For this review, take the finished solid that the model builds, in its own axes (mm). Round coordinates to 2 decimals unless told otherwise and drop trailing zeros. Write each loop counter-clockwise with the first axis right and the second up, starting at its lowest first coordinate (ties: lowest second). Pieces come first, ordered by that corner, then holes. Notation, with made-up numbers: (42.5, 59.5) -> (92.5, 59.5) arc R28 cw to (92.5, 78.5) -> close; hole circle Ø4 at (-3, -30). An arc over 180 degrees is marked (long way). Answer in a Markdown table with one row per item. Add a question column.
```python
from build123d import *

# Parameters (mm, degrees)
SKETCH1_W                                   = 50.5
SKETCH1_H                                   = 51.5
SKETCH1_R                                   = 1.775
BOSS_EXTRUDE1_DEPTH                         = 3.5
CSK_FOR_10_FLAT_HEAD_SOCKET_CAP_SCR_2_COUNT = 2
CSK_FOR_10_FLAT_HEAD_SOCKET_CAP_SCR_2_PITCH = 20


with BuildPart() as part:
    # Sketch1 → Boss-Extrude1 (new body)
    with BuildSketch(Plane(origin=(0, 0, 0), x_dir=(1, 0, 0), z_dir=(0, 1, 0))):
        Rectangle(SKETCH1_W, SKETCH1_H)
        with Locations(Location((-19.475, 19.975, 0), (0, 0, 270))):
            Circle(SKETCH1_R, mode=Mode.SUBTRACT)
        with Locations(Location((19.475, 19.975, 0), (0, 0, 270))):
            Circle(SKETCH1_R, mode=Mode.SUBTRACT)
        with Locations(Location((19.475, -19.975, 0), (0, 0, 270))):
            Circle(SKETCH1_R, mode=Mode.SUBTRACT)
        with Locations(Location((-19.475, -19.975, 0), (0, 0, 270))):
            Circle(SKETCH1_R, mode=Mode.SUBTRACT)
    extrude(amount=BOSS_EXTRUDE1_DEPTH)

    # Sketch4 → CSK for #10 Flat Head Socket Cap Screw1 (revolve, cut)
    with BuildSketch(Plane(origin=(0, 3.5, -10), x_dir=(0, 0, 1), z_dir=(1, 0, 0))):
        Polygon((0, 0), (0, 3.5), (2.5527, 3.5), (2.5527, 3.068032542), (5.2197, 0), align=None)
    csk_for_10_flat_head_socket_cap_screw1 = revolve(axis=Axis((0, 9.85, -10), (0, -1, 0)), mode=Mode.SUBTRACT)

    # CSK for _10 Flat Head Socket Cap Scr 2: CSK for #10 Flat Head Socket Cap Screw1 ×2
    with Locations(*[(0, 0, i * CSK_FOR_10_FLAT_HEAD_SOCKET_CAP_SCR_2_PITCH) for i in range(1, CSK_FOR_10_FLAT_HEAD_SOCKET_CAP_SCR_2_COUNT)]):
        add(csk_for_10_flat_head_socket_cap_screw1, mode=Mode.SUBTRACT)


solid = part.part
```
1. We need section B-B (x = 0). Write out the cut boundary in (y, z).
2. We need section A-A (z = -10). Write out the cut boundary in (x, y), plus the area to 3 significant figures.
3. We need section C-C (z = 20). Write out the cut boundary in (x, y), plus the area to 3 significant figures.
4. The part is to be moulded in two halves that separate along Z. For faces 1 (the flat face through (0, 2, 25.75)), 2 (the flat face through (0, 0, 0)), 3 (the cylindrical face through (-0.767, 0.219, 12.435)), say which applies: pulls with the +Z half, pulls with the -Z half, needs draft (parallel to the pull), parting line crosses it, or undercut.
5. Clearance check with a flat-ended pin moving along its axis: pin 1 Ø6 at (x, z) = (0, 10) entering from +Y. State where the tip first meets the part, or that it passes through.
6. For L1, parallel to X at y = 1.8, z = -20; L2, parallel to Z at x = 0, y = 0.25; L3, parallel to X at y = 2.2, z = 20.5, list the stretches that pass through material, from the lowest coordinate up. Write a range as [from, to].
7. We need section D-D (y = 2.1). Write out the cut boundary in (x, z) (3 decimals).
Response:
| question | item | result |
|---|---|---|
| 1 | outline | (0, -25.75) -> (3.5, -25.75) -> (3.5, -15.22) -> (0.43, -12.55) -> (0, -12.55) -> close; (0, -7.45) -> (0.43, -7.45) -> (3.5, -4.78) -> (3.5, 4.78) -> (0.43, 7.45) -> (0, 7.45) -> close; (0, 12.55) -> (0.43, 12.55) -> (3.5, 15.22) -> (3.5, 25.75) -> (0, 25.75) -> close |
| 2 | outline | (-25.25, 0) -> (-2.55, 0) -> (-2.55, 0.43) -> (-5.22, 3.5) -> (-25.25, 3.5) -> close; (2.55, 0) -> (25.25, 0) -> (25.25, 3.5) -> (5.22, 3.5) -> (2.55, 0.43) -> close |
| 2 | area | 151 mm2 |
| 3 | outline | (-25.25, 0) -> (-21.25, 0) -> (-21.25, 3.5) -> (-25.25, 3.5) -> close; (-17.7, 0) -> (17.7, 0) -> (17.7, 3.5) -> (-17.7, 3.5) -> close; (21.25, 0) -> (25.25, 0) -> (25.25, 3.5) -> (21.25, 3.5) -> close |
| 3 | area | 152 mm2 |
| 4 | face 1 | pulls with the +Z half |
| 4 | face 2 | needs draft |
| 4 | face 3 | undercut |
| 5 | pin 1 | y = 0.95 |
| 6 | L1 | [-25.25, -21.25], [-17.7, 17.7], [21.25, 25.25] |
| 6 | L2 | [-25.75, -12.55], [-7.45, 7.45], [12.55, 25.75] |
| 6 | L3 | [-25.25, -21.17], [-17.78, 17.78], [21.17, 25.25] |
| 7 | outline | (-25.25, -25.75) -> (25.25, -25.75) -> (25.25, 25.75) -> (-25.25, 25.75) -> close; hole circle Ø3.55 at (-19.475, -19.975); hole circle Ø3.55 at (-19.475, 19.975); hole circle Ø8.005 at (0, -10); hole circle Ø8.005 at (0, 10); hole circle Ø3.55 at (19.475, -19.975); hole circle Ø3.55 at (19.475, 19.975) |
